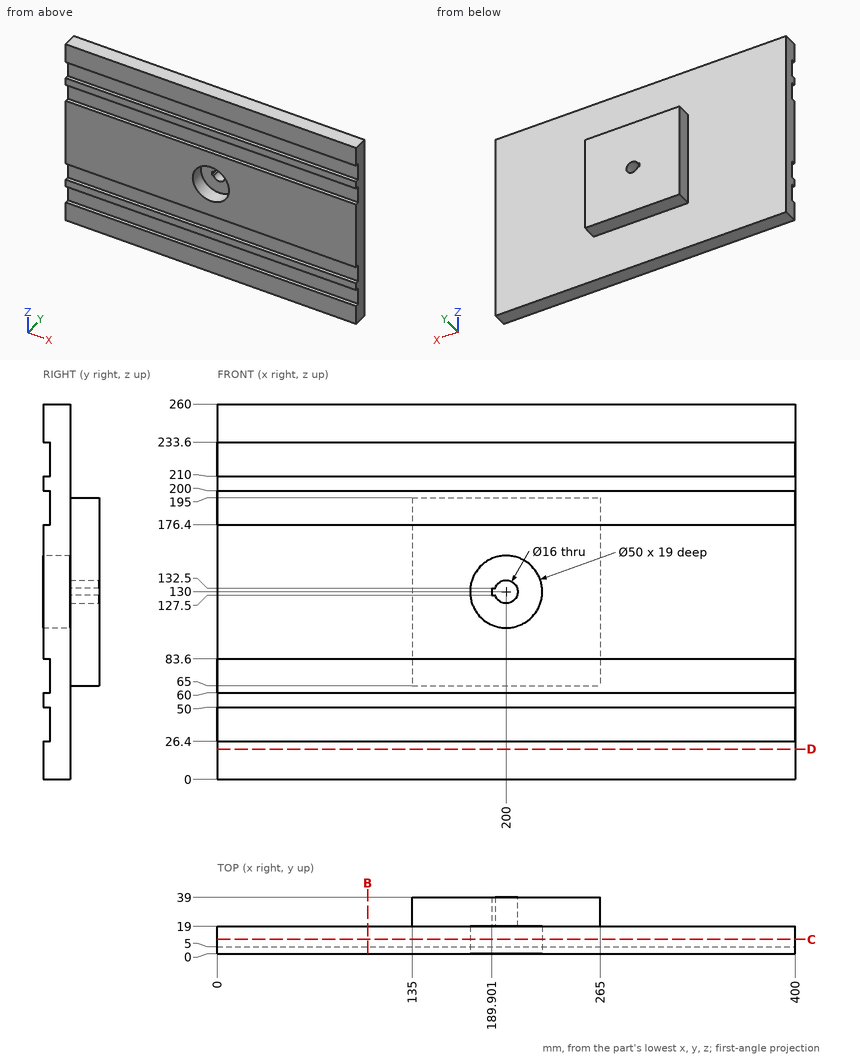
For this review, use the dimensioned drawing (mm, ordinates from the lowest corner) and the shaded views. Coordinates: 2 decimals unless noted, no trailing zeros. Loops run counter-clockwise (first coordinate to the right, second up) from the corner with the lowest first, then second, coordinate; pieces in that order, holes last. Notation, with made-up numbers: (52, 29) -> (97, 29) arc R17 ccw to (97, 36) -> close; hole circle Ø9 at (40, -7). An arc over 180 degrees is marked (long way). Return JSON: item names as keys, results as strings. Group by question number.
(1) To check wall thickness, follow L1, parallel to Z at x = 360.5, y = 4.5; L2, parallel to Z at x = 200, y = 32; L3, parallel to X at y = 13, z = 130. State the ranges of each line that lie inside material, in increasing order.
(2) Consider section C-C, the plane y = 10. Give the boundary of the cut face in (x, z), plus the area to 3 significant figures.
(3) Consider section D-D, the plane z = 21. Give the boundary of the cut face in (x, y), plus the area to 3 significant figures.
(4) For pin 1 Ø10 at (x, z) = (116.5, 115) entering from +Y; pin 2 Ø4 at (y, z) = (30, 129.5) entering from +X; pin 3 Ø16 at (y, z) = (27.5, 121.5) entering from -X, all flat-tipped, find the tip position at first contact; note any pin that passes through.
(5) Consider section B-B, the plane x = 104. Give the boundary of the cut face in (y, z).
Results below:
{
 "1": {"L1": "z = 0 to 26.4, 50 to 60, 83.6 to 176.4, 200 to 210, 233.6 to 260", "L2": "z = 65 to 122, 138 to 195", "L3": "x = 0 to 175, 225 to 400"},
 "2": {"outline": "(0, 0) -> (400, 0) -> (400, 260) -> (0, 260) -> close; hole circle Ø50 at (200, 130)", "area": "102,000 mm2"},
 "3": {"outline": "(0, 0) -> (400, 0) -> (400, 19) -> (0, 19) -> close", "area": "7,600 mm2"},
 "4": {"pin 1": "stops at y = 19", "pin 2": "stops at x = 265", "pin 3": "stops at x = 135"},
 "5": {"outline": "(0, 0) -> (19, 0) -> (19, 260) -> (0, 260) -> (0, 233.6) -> (5, 233.6) -> (5, 210) -> (0, 210) -> (0, 200) -> (5, 200) -> (5, 176.4) -> (0, 176.4) -> (0, 83.6) -> (5, 83.6) -> (5, 60) -> (0, 60) -> (0, 50) -> (5, 50) -> (5, 26.4) -> (0, 26.4) -> close"}
}
